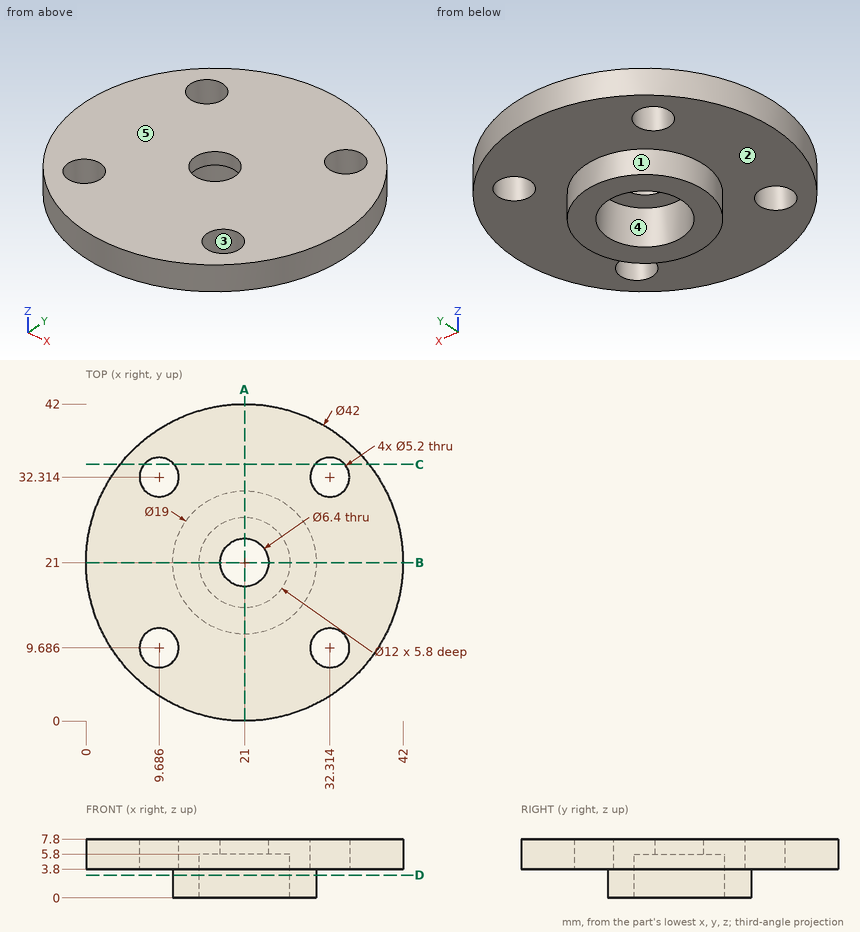
Drawing for the job (mm, zero at the part's lowest x, y, z). A direction names the side the tool comes from. Round coordinates to 2 decimals unless told otherwise and drop trailing zeros. Write each loop counter-clockwise with the first axis right and the second up, starting at its lowest first coordinate (ties: lowest second). Pieces come first, ordered by that corner, then holes. Notation, with made-up numbers: (-10.75, 64) - (31.25, 64) arc R28 cw to (31.25, 96) - close; hole circle Ø1 at (-4.5, 39.5). An arc over 180 degrees is marked (long way). Return JSON: item names as keys, results as strings. Group by question number.
Item 1: Flat gauge pins, fed straight in: pin 1 Ø4.5 at (x, y) = (9.69, 32.31) entering from +Z; pin 2 Ø1 at (x, z) = (28, 6.5) entering from -Y; pin 3 Ø1.5 at (x, z) = (37, 3.5) entering from -Y; pin 4 Ø7 at (x, y) = (32.31, 9.69) entering from -Z. Where does each tip first touch, or does it go through?
Item 2: 3-axis set-ups, long thin cutter, end or side, ignore diameter. For the marked faces 4 and 5: which of +Z, -Z, +X, -X, +Y, -Y reach the whole face in a straight line?
Item 3: Probe probe 1 along Z at (x, y) = (9.5, 23.5); probe 2 along Y at (x, z) = (21, 7.2); probe 3 along X at (y, z) = (12, 5) (1 decimal). List the from-to ranges inside material, lowest first.
Item 4: Mould opens along Y. For the marked faces 1, 2 and 3 say: +Y half, -Y half, draft (parallel to the pull), parting line (faces both ways), or undercut.
Item 5: Band-saw the part on A-A on x = 21. List the corners of the cut face in (y, z), plus the area to 3 significant figures.
Item 6: Band-saw the part on C-C on y = 34. List the corners of the cut face in (x, z) (1 decimal).
Item 7: Band-saw the part on D-D on z = 3. List the corners of the cut face in (x, y), plus the area to 3 significant figures.
Resolved:
{
 "1": {"pin 1": "passes through", "pin 2": "stops at y = 1.03", "pin 3": "stops at y = 6.63", "pin 4": "stops at z = 3.8"},
 "2": {"face 4": "-Z", "face 5": "+Z, +X, -X, +Y, -Y"},
 "3": {"probe 1": "z = 3.8 to 7.8", "probe 2": "y = 0 to 17.8, 24.2 to 42", "probe 3": "x = 2 to 8.5, 10.9 to 31.1, 33.5 to 40"},
 "4": {"face 1": "parting line", "face 2": "draft", "face 3": "undercut"},
 "5": {"outline": "(0, 3.8) - (11.5, 3.8) - (11.5, 0) - (15, 0) - (15, 5.8) - (17.8, 5.8) - (17.8, 7.8) - (0, 7.8) - close; (24.2, 5.8) - (27, 5.8) - (27, 0) - (30.5, 0) - (30.5, 3.8) - (42, 3.8) - (42, 7.8) - (24.2, 7.8) - close", "area": "158 mm²"},
 "6": {"outline": "(4.5, 3.8) - (7.7, 3.8) - (7.7, 7.8) - (4.5, 7.8) - close; (11.7, 3.8) - (30.3, 3.8) - (30.3, 7.8) - (11.7, 7.8) - close; (34.3, 3.8) - (37.5, 3.8) - (37.5, 7.8) - (34.3, 7.8) - close"},
 "7": {"outline": "circle Ø19 at (21, 21); hole circle Ø12 at (21, 21)", "area": "170 mm²"}
}
